```python
from build123d import *

# Parameters (mm, degrees)
F4_DEPTH     = 5.08
F5_SIZE2     = 5.07999
F5_SIZE      = 5.07999
F6_T1_DEPTH  = 83.8598569958
F6_T3_DEPTH  = 84.6306377444
F6_T8_DEPTH  = 42.5046669686
F6_T13_DEPTH = 41.8031738059


# Not quite as in the source:
# - a fillet or chamfer that OpenCascade refuses, or shapes differently, is made with other operations: its cross-section is extruded or revolved along the edge and cut away or added
# - a fillet or chamfer is up to 0.001 mm smaller than in the source, because OpenCascade refuses the exact size
# - the program builds the solid bodies; features that only make, move or delete a surface that nothing else refers to are left out


with BuildPart() as f4:
    # F0 (on Top) → F4 (new body)
    with BuildSketch(Plane.XY):
        Polygon((-2.3713386618, 16.203770414), (-51.0019175708, 47.3164618015), (-19.3783510476, -1.9021694316), (-3.9232242852, -4.51765256), (18.5309383262, -26.9124830378), (23.3981461688, -22.2631122398), (0, 0), align=None)
    extrude(amount=F4_DEPTH)

    # F5 (size 5.08 and 5.08 in the source; OpenCascade refuses exactly that, so slightly less here)
    f5_edges = [f4.edges().sort_by_distance(p)[0] for p in [
        (-11.650788, -3.209911, 0),
        (-35.190134, 22.707146, 0),
        (-26.686628, 31.760116, 0),
        (-1.185669, 8.101885, 0),
    ]]
    chamfer(f5_edges, length=F5_SIZE, length2=F5_SIZE2)

    # F6: chamfer of 5.08 on 4 edges, made by hand

    # F6_s2 → F6_t1 (cut)
    with BuildSketch(Plane(origin=(1.9661453214, -1.2578931606, 0), x_dir=(0, 0, 1), z_dir=(-0.8423569488, 0.5389200041, 0))):
        Polygon((0, 12.3713967634), (5.08, 7.2913967634), (5.08, 12.3713967634), align=None)
    extrude(amount=F6_T1_DEPTH, mode=Mode.SUBTRACT)

    # F6_s4 → F6_t3 (cut)
    with BuildSketch(Plane(origin=(-43.4826566064, 67.6760111474, 0), x_dir=(0, 0, 1), z_dir=(0.5405521777, -0.8413104915, 0))):
        Polygon((5.08, 12.2514318739), (0, 17.3314318739), (5.08, 17.3314318739), align=None)
    extrude(amount=F6_T3_DEPTH, mode=Mode.SUBTRACT)


with BuildPart() as f6_tool6:
    # F6_s7 → F6_t8 (new body)
    with BuildSketch(Plane(origin=(1.8917212496, -12.9264610367, 0), x_dir=(0, 0, 1), z_dir=(-0.1448024793, 0.9894605813, 0))):
        Polygon((0, 0), (5.08, -5.08), (5.08, 0), align=None)
    extrude(amount=F6_T8_DEPTH)

    split(bisect_by=Plane(origin=(0, 0, 0), x_dir=(0, 0, 1), z_dir=(0.6893167986, 0.7244600411, 0)), keep=Keep.TOP)


with BuildPart() as f4_1:
    add(f4.part)

    # F6_t5: cut F6_tool6
    add(f6_tool6.part, mode=Mode.SUBTRACT)


with BuildPart() as f6_tool11:
    # F6_s12 → F6_t13 (new body)
    with BuildSketch(Plane(origin=(-31.4068834176, 5.3150113201, 0), x_dir=(0, 0, 1), z_dir=(0.985980884, -0.1668583122, 0))):
        Polygon((5.08, 0.0289416476), (0, 5.1089416476), (5.08, 5.1089416476), align=None)
    extrude(amount=F6_T13_DEPTH)

    split(bisect_by=Plane(origin=(-4.2152403692, -4.2264080896, 0), x_dir=(0, 0, 1), z_dir=(-0.7061707096, -0.7080416152, 0)), keep=Keep.TOP)


with BuildPart() as f4_2:
    add(f4_1.part)

    # F6_t10: cut F6_tool11
    add(f6_tool11.part, mode=Mode.SUBTRACT)


solid = f4_2.part
```
The listing builds one solid part. Answer for the finished solid, in the listing's coordinates (mm). Round coordinates to 2 decimals unless told otherwise and drop trailing zeros. Loops run counter-clockwise (first coordinate to the right, second up) from the corner with the lowest first, then second, coordinate; pieces in that order, holes last.
Q1. Section A-A, the plane z = 3.8 is taken. Determine the outline of the cut face in (x, y).
Q2. Section D-D, the plane x = -30 is taken. Determine the outline of the cut face in (y, z), then the cut area to 3 significant figures.
Q3. Section C-C, the plane y = 16 is taken. Determine the outline of the cut face in (x, z).
Q4. Section B-B, the plane x = -8 is taken. Determine the outline of the cut face in (y, z).
Q5. Find the intervals of material crossed by line 1 (Z direction, x = -24, y = 26); line 2 (X direction, y = 29, z = 0.75); line 3 (X direction, y = -19.5, z = 1.95), in increasing order.
Q6. Given pin 1 Ø1 at (y, z) = (11.5, 2.5) entering from -X; pin 2 Ø1.5 at (x, z) = (1, 2.5) entering from +Y; pin 3 Ø1 at (x, z) = (-15, 4.5) entering from -Y, each flat-ended and moving along its own axis, determine where each tip first touches the part or whether it passes through.
Completed:
1. outline: (-38.41, 34.75) - (-17.09, 1.56) - (-8.58, 0.12) - (18.53, -26.91) - (23.4, -22.26) - (-4.46, 4.25) - (-5.88, 13.94) - close
2. outline: (19.33, 2.54) - (24.03, 0) - (27.85, 0) - (30.86, 2.54) - (27.85, 5.08) - (24.03, 5.08) - close
2. area: 39.0 mm2
3. outline: (-27.86, 2.54) - (-24.84, 0) - (-11.48, 0) - (-6.77, 2.54) - (-11.48, 5.08) - (-24.84, 5.08) - close
4. outline: (-1.25, 2.54) - (-0.45, 1.75) - (-0.45, 0) - (13.77, 0) - (16.79, 2.54) - (13.77, 5.08) - (-0.45, 5.08) - (-0.45, 3.33) - close
5. line 1: z = 1.68 to 3.4
5. line 2: x = -34.09 to -30.41
5. line 3: x = 11.1 to 20.49
6. pin 1: stops at x = -25.29
6. pin 2: stops at y = -0.24
6. pin 3: stops at y = 1.41
